For this review, take the finished solid that the model builds, in its own axes (mm). Give positions to 0.01 mm unless a question says otherwise; leave off trailing zeros. Loops run counter-clockwise (first coordinate to the right, second up) from the corner with the lowest first, then second, coordinate; pieces in that order, holes last. Notation, with made-up numbers: (86.25, 70.5) - (131.25, 70.5) arc R37 cw to (131.25, 107.5) - close; hole circle Ø3 at (-4.5, 33). An arc over 180 degrees is marked (long way). Answer as CSV lines item,"result".
from build123d import *

# Parameters (mm, degrees)
CYLINDER425_R               = 1.6
CYLINDER425_DEPTH           = 15
CYLINDER425_PLACEMENT_ANGLE = 3
CYLINDER428_R               = 1.6
CYLINDER428_DEPTH           = 15
CYLINDER428_PLACEMENT_ANGLE = 3
CYLINDER426_R               = 1.6
CYLINDER426_DEPTH           = 15
CYLINDER426_PLACEMENT_ANGLE = 3
CYLINDER427_R               = 1.6
CYLINDER427_DEPTH           = 15
CYLINDER427_PLACEMENT_ANGLE = 3
CYLINDER422_R               = 3
CYLINDER422_DEPTH           = 2
CYLINDER422_PLACEMENT_ANGLE = 3
CYLINDER423_R               = 3
CYLINDER423_DEPTH           = 2
CYLINDER423_PLACEMENT_ANGLE = 3
CYLINDER424_R               = 3
CYLINDER424_DEPTH           = 2
CYLINDER424_PLACEMENT_ANGLE = 3
CYLINDER421_R               = 3
CYLINDER421_DEPTH           = 2
CYLINDER421_PLACEMENT_ANGLE = 3
BOX289_W                    = 62.5
BOX289_H                    = 119.5
BOX289_DEPTH                = 2.5
BOX288_W                    = 74.5
BOX288_H                    = 99.5
BOX288_DEPTH                = 2.5
CHAMFER028_SIZE             = 0.5
CHAMFER028_PLACEMENT_ANGLE  = 3


with BuildPart() as cylinder560:
    # Cylinder425 → Cylinder425 (new body)
    with BuildSketch(Plane.XY):
        Circle(CYLINDER425_R)
    extrude(amount=CYLINDER425_DEPTH)


with BuildPart() as cylinder560_1:
    # Cylinder425 placement: moved
    add(cylinder560.part.moved(Location((380.5, -14, -52))).rotate(Axis((380.5, -14, -52), (0, -1, 0)), CYLINDER425_PLACEMENT_ANGLE))


with BuildPart() as fusion380:
    # Cylinder428 → Cylinder428 (new body)
    with BuildSketch(Plane.XY):
        Circle(CYLINDER428_R)
    extrude(amount=CYLINDER428_DEPTH)


with BuildPart() as fusion380_1:
    # Cylinder428 placement: moved
    add(fusion380.part.moved(Location((311.5, -14, -56))).rotate(Axis((311.5, -14, -56), (0, -1, 0)), CYLINDER428_PLACEMENT_ANGLE))

    # Fusion380: union Cylinder560
    add(cylinder560_1.part)


with BuildPart() as cylinder561:
    # Cylinder426 → Cylinder426 (new body)
    with BuildSketch(Plane.XY):
        Circle(CYLINDER426_R)
    extrude(amount=CYLINDER426_DEPTH)


with BuildPart() as cylinder561_1:
    # Cylinder426 placement: moved
    add(cylinder561.part.moved(Location((380.5, -14, -52))).rotate(Axis((380.5, -14, -52), (0, -1, 0)), CYLINDER426_PLACEMENT_ANGLE))


with BuildPart() as fusion379:
    # Cylinder427 → Cylinder427 (new body)
    with BuildSketch(Plane.XY):
        Circle(CYLINDER427_R)
    extrude(amount=CYLINDER427_DEPTH)


with BuildPart() as fusion379_1:
    # Cylinder427 placement: moved
    add(fusion379.part.moved(Location((311.5, -14, -56))).rotate(Axis((311.5, -14, -56), (0, -1, 0)), CYLINDER427_PLACEMENT_ANGLE))

    # Fusion378: union Cylinder561
    add(cylinder561_1.part)


with BuildPart() as fusion379_2:
    # Fusion378 placement: moved
    add(fusion379_1.part.moved(Location((0, 90, 0))))

    # Fusion379: union Fusion380
    add(fusion380_1.part)


with BuildPart() as cylinder557:
    # Cylinder422 → Cylinder422 (new body)
    with BuildSketch(Plane.XY):
        Circle(CYLINDER422_R)
    extrude(amount=CYLINDER422_DEPTH)


with BuildPart() as cylinder557_1:
    # Cylinder422 placement: moved
    add(cylinder557.part.moved(Location((380.5, -14, -52))).rotate(Axis((380.5, -14, -52), (0, -1, 0)), CYLINDER422_PLACEMENT_ANGLE))


with BuildPart() as fusion376:
    # Cylinder423 → Cylinder423 (new body)
    with BuildSketch(Plane.XY):
        Circle(CYLINDER423_R)
    extrude(amount=CYLINDER423_DEPTH)


with BuildPart() as fusion376_1:
    # Cylinder423 placement: moved
    add(fusion376.part.moved(Location((311.5, -14, -56))).rotate(Axis((311.5, -14, -56), (0, -1, 0)), CYLINDER423_PLACEMENT_ANGLE))

    # Fusion376: union Cylinder557
    add(cylinder557_1.part)


with BuildPart() as cylinder559:
    # Cylinder424 → Cylinder424 (new body)
    with BuildSketch(Plane.XY):
        Circle(CYLINDER424_R)
    extrude(amount=CYLINDER424_DEPTH)


with BuildPart() as cylinder559_1:
    # Cylinder424 placement: moved
    add(cylinder559.part.moved(Location((380.5, -14, -52))).rotate(Axis((380.5, -14, -52), (0, -1, 0)), CYLINDER424_PLACEMENT_ANGLE))


with BuildPart() as fusion381:
    # Cylinder421 → Cylinder421 (new body)
    with BuildSketch(Plane.XY):
        Circle(CYLINDER421_R)
    extrude(amount=CYLINDER421_DEPTH)


with BuildPart() as fusion381_1:
    # Cylinder421 placement: moved
    add(fusion381.part.moved(Location((311.5, -14, -56))).rotate(Axis((311.5, -14, -56), (0, -1, 0)), CYLINDER421_PLACEMENT_ANGLE))

    # Fusion377: union Cylinder559
    add(cylinder559_1.part)


with BuildPart() as fusion381_2:
    # Fusion377 placement: moved
    add(fusion381_1.part.moved(Location((0, 90, 0))))

    # Fusion375: union Fusion376
    add(fusion376_1.part)

    # Fusion381: union Fusion379
    add(fusion379_2.part)


with BuildPart() as cube369:
    # Box289 → Box289 (new body)
    with BuildSketch(Plane(origin=(8.75, -23.75, -0.5), x_dir=(1, 0, 0), z_dir=(0, 0, 1))):
        with Locations((31.25, 59.75)):
            Rectangle(BOX289_W, BOX289_H)
    extrude(amount=BOX289_DEPTH)


with BuildPart() as battery_box_wide_closure:
    # Box288 → Box288 (new body)
    with BuildSketch(Plane(origin=(2.75, -13.75, -0.5), x_dir=(1, 0, 0), z_dir=(0, 0, 1))):
        with Locations((37.25, 49.75)):
            Rectangle(BOX288_W, BOX288_H)
    extrude(amount=BOX288_DEPTH)

    # Fusion371: union Cube369
    add(cube369.part)

    # Chamfer028
    chamfer028_edges = [battery_box_wide_closure.edges().sort_by_distance(p)[0] for p in [
        (2.75, 36, 2),
        (5.75, -13.75, 2),
        (5.75, 85.75, 2),
        (8.75, -18.75, 2),
        (8.75, 90.75, 2),
        (40, -23.75, 2),
        (40, 95.75, 2),
        (71.25, -18.75, 2),
        (71.25, 90.75, 2),
        (74.25, 85.75, 2),
        (77.25, 36, 2),
        (74.25, -13.75, 2),
    ]]
    chamfer(chamfer028_edges, length=CHAMFER028_SIZE)


with BuildPart() as battery_box_wide_closure_1:
    # Chamfer028 placement: moved
    add(battery_box_wide_closure.part.moved(Location((306, -5, -54.5))).rotate(Axis((306, -5, -54.5), (0, -1, 0)), CHAMFER028_PLACEMENT_ANGLE))

    # Cut291: cut Fusion381
    add(fusion381_2.part, mode=Mode.SUBTRACT)


solid = battery_box_wide_closure_1.part
1) Wall thickness on line 1 (Y direction, x = 312, z = -52.5); line 2 (Z direction, x = 334, y = 49); line 3 (Z direction, x = 351, y = -10.5): over which ranges is each line inside the solid? List them lowest first. Write a range as from..to.
From the geometry:
line 1,"y = -18.57..-15.45, -12.55..74.55, 77.45..80.57"
line 2,"z = -53.53..-51.03"
line 3,"z = -52.64..-50.14"
2) Consider section A-A on y = 11.5. Write out the cut boundary in (x, z).
From the geometry:
outline,"(308.67, -52.86) - (308.77, -54.86) - (383.17, -50.96) - (383.07, -48.96) - (382.54, -48.49) - (309.14, -52.33) - close"
3) Insertion check: P1, Ø1.2, axis at x = 380.5, z = -49.5, coming from the -Y side; P2, Ø1, axis at x = 367.5, y = 4, coming from the -Z side; P3, Ø3, axis at y = 61.5, z = -51, coming from the -X side. Each pin has a flat end and moves straight along its axis. Give the tip position at first contact, or say it passes through.
From the geometry:
P1,"stops at y = -18.75"
P2,"stops at z = -51.8"
P3,"stops at x = 308.99"
4) Consider section B-B on x = 336. Write out the cut boundary in (y, z).
From the geometry:
outline,"(-28.75, -53.43) - (90.75, -53.43) - (90.75, -51.43) - (90.25, -50.93) - (-28.25, -50.93) - (-28.75, -51.43) - close"
5) Draft analysis for pull direction X (two halves, no side actions). For faces 1 (the flat face through (380, -18.75, -50)), 2 (the flat face through (345.417, 90.504, -50.685)), 3 (the cylindrical face through (314.41, 75.89, -54.21)), state which applies: pulls with the +X half, pulls with the -X half, needs draft (parallel to the pull), parting line crosses it, or undercut.
From the geometry:
face 1,"needs draft"
face 2,"pulls with the -X half"
face 3,"undercut"
